Check sheet for the modelled part. Datum: model origin and axes. Units: mm. Face numbers are marked on the shaded views. A direction names the side the tool comes from. Give positions to 0.01 mm unless a question says otherwise; leave off trailing zeros. Loops run counter-clockwise (first coordinate to the right, second up) from the corner with the lowest first, then second, coordinate; pieces in that order, holes last. Notation, with made-up numbers: (73.25, 79) - (120.25, 79) arc R19 ccw to (120.25, 90) - close; hole circle Ø9 at (8.25, -36.5). An arc over 180 degrees is marked (long way). Use one line per item in the form item = value.
from build123d import *

# Parameters (mm, degrees)
SKETCH_1_R          = 4.1
SKETCH_1_R_2        = 1.6
EXTRUDE_1_DEPTH     = 7.5
CUT_EXTRUDE_1_DEPTH = 2.5
SKETCH_4_R          = 3.6
SKETCH_4_R_2        = 1.6
EXTRUDE_2_DEPTH     = 20
SKETCH_5_R          = 7
SKETCH_5_R_2        = 1.6
EXTRUDE_3_DEPTH     = 10
CUT_EXTRUDE_START   = -6.5
CUT_EXTRUDE_2_DEPTH = 6.5
SKETCH_7_R          = 1.6
CUT_EXTRUDE_3_DEPTH = 86.794813363
CHAMFER_1_SIZE      = 1
CHAMFER_1_SIZE_2    = 22
SKETCH_9_R          = 3.35
CUT_EXTRUDE_4_DEPTH = 3
SKETCH_11_R         = 3.35
CUT_EXTRUDE_5_DEPTH = 3


with BuildPart() as part:
    # 草图1 → 凸台-拉伸1 (new body)
    with BuildSketch(Plane.XY):
        Polygon((0, 11.5), (0, 4.5), (0.416202301, 4.5), (28, 4.5), (28, 0), (47, 0), (47, 4.5), (75, 4.5), (75, 18.5), (47, 18.5), (47, 23.5), (28, 23.5), (28, 18.5), (0, 18.5), align=None)
        with Locations((37.5, 11.5)):
            Circle(SKETCH_1_R, mode=Mode.SUBTRACT)
        with Locations((67.5, 11.5)):
            Circle(SKETCH_1_R_2, mode=Mode.SUBTRACT)
        with Locations((32.500024738, 3.227756818)):
            Circle(SKETCH_1_R_2, mode=Mode.SUBTRACT)
        with Locations((42.5, 3.25)):
            Circle(SKETCH_1_R_2, mode=Mode.SUBTRACT)
        with Locations((42.5, 19.75)):
            Circle(SKETCH_1_R_2, mode=Mode.SUBTRACT)
        with Locations((32.500024738, 19.75)):
            Circle(SKETCH_1_R_2, mode=Mode.SUBTRACT)
        with Locations((7.5, 11.5)):
            Circle(SKETCH_1_R_2, mode=Mode.SUBTRACT)
        with Locations((52.370486737, 11.554033831)):
            Circle(SKETCH_1_R_2, mode=Mode.SUBTRACT)
        with Locations((22.5, 11.5)):
            Circle(SKETCH_1_R_2, mode=Mode.SUBTRACT)
    extrude(amount=EXTRUDE_1_DEPTH)

    # 草图2 → 切除-拉伸1 (cut)
    with BuildSketch(Plane(origin=(0, 0, 0), x_dir=(-1, 0, 0), z_dir=(0, 0, -1))):
        Polygon((-38.862693304, 19.75), (-40.681346652, 22.9), (-44.318653348, 22.9), (-46.137306696, 19.75), (-44.318653348, 16.6), (-40.681346652, 16.6), align=None)
        Polygon((-28.862718042, 19.75), (-30.68137139, 22.9), (-34.318678086, 22.9), (-36.137331434, 19.75), (-34.318678086, 16.6), (-30.68137139, 16.6), align=None)
        Polygon((-38.862693304, 3.25), (-40.681346652, 6.4), (-44.318653348, 6.4), (-46.137306696, 3.25), (-44.318653348, 0.1), (-40.681346652, 0.1), align=None)
        Polygon((-28.862718042, 3.227756818), (-30.68137139, 6.377756818), (-34.318678086, 6.377756818), (-36.137331434, 3.227756818), (-34.318678086, 0.077756818), (-30.68137139, 0.077756818), align=None)
        Polygon((-63.862693304, 11.5), (-65.681346652, 14.65), (-69.318653348, 14.65), (-71.137306696, 11.5), (-69.318653348, 8.35), (-65.681346652, 8.35), align=None)
        Polygon((-3.862693304, 11.5), (-5.681346652, 14.65), (-9.318653348, 14.65), (-11.137306696, 11.5), (-9.318653348, 8.35), (-5.681346652, 8.35), align=None)
    extrude(amount=-CUT_EXTRUDE_1_DEPTH, mode=Mode.SUBTRACT)

    # 草图4 → 凸台-拉伸2 (add)
    # profile 1 of 2: a face of its own
    with BuildSketch(Plane.XY.offset(7.5)):
        with Locations(Location((7.5, 11.5, 0), (0, 0, 180))):
            Circle(SKETCH_4_R)
        with Locations(Location((7.5, 11.5, 0), (0, 0, 180))):
            Circle(SKETCH_4_R_2, mode=Mode.SUBTRACT)
    # profile 2 of 2: a face of its own
    with BuildSketch(Plane.XY.offset(7.5)):
        with Locations(Location((67.5, 11.5, 0), (0, 0, 180))):
            Circle(SKETCH_4_R)
        with Locations(Location((67.5, 11.5, 0), (0, 0, 180))):
            Circle(SKETCH_4_R_2, mode=Mode.SUBTRACT)
    extrude(amount=EXTRUDE_2_DEPTH)

    # 草图5 → 凸台-拉伸3 (add)
    # profile 1 of 2: a face of its own
    with BuildSketch(Plane.XY.offset(27.5)):
        with Locations((7.5, 11.5)):
            Circle(SKETCH_5_R)
        with Locations(Location((7.5, 11.5, 0), (0, 0, 180))):
            Circle(SKETCH_5_R_2, mode=Mode.SUBTRACT)
    # profile 2 of 2: a face of its own
    with BuildSketch(Plane.XY.offset(27.5)):
        with Locations((67.5, 11.5)):
            Circle(SKETCH_5_R)
        with Locations(Location((67.5, 11.5, 0), (0, 0, 180))):
            Circle(SKETCH_5_R_2, mode=Mode.SUBTRACT)
    extrude(amount=EXTRUDE_3_DEPTH)

    # 草图6 → 切除-拉伸2 (cut)
    with BuildSketch(Plane.XY.offset(37.5).offset(CUT_EXTRUDE_START)):
        with BuildLine():
            Line((1.5, 7.894448725), (1.5, 15.105551275))
            ThreePointArc((1.5, 15.105551275), (0.5, 11.5), (1.5, 7.894448725))
        make_face()
        with BuildLine():
            Line((73.5, 15.105551275), (73.5, 7.894448725))
            ThreePointArc((73.5, 7.894448725), (74.5, 11.5), (73.5, 15.105551275))
        make_face()
        with BuildLine():
            Line((3.5, 5.755437353), (3.5, 17.244562647))
            ThreePointArc((3.5, 17.244562647), (7.5, 18.5), (11.5, 17.244562647))
            Line((11.5, 17.244562647), (11.5, 5.755437353))
            ThreePointArc((11.5, 5.755437353), (7.5, 4.5), (3.5, 5.755437353))
        make_face()
        with BuildLine():
            Line((71.5, 7.894448725), (71.5, 17.244562647))
            ThreePointArc((71.5, 17.244562647), (67.5, 18.5), (63.5, 17.244562647))
            Line((63.5, 17.244562647), (63.5, 5.755437353))
            ThreePointArc((63.5, 5.755437353), (67.5, 4.5), (71.5, 5.755437353))
            Line((71.5, 5.755437353), (71.5, 7.894448725))
        make_face()
        with BuildLine():
            Line((13.5, 15.105551275), (13.5, 7.894448725))
            ThreePointArc((13.5, 7.894448725), (14.5, 11.5), (13.5, 15.105551275))
        make_face()
        with BuildLine():
            Line((61.5, 7.894448725), (61.5, 15.105551275))
            ThreePointArc((61.5, 15.105551275), (60.5, 11.5), (61.5, 7.894448725))
        make_face()
    extrude(amount=CUT_EXTRUDE_2_DEPTH, mode=Mode.SUBTRACT)

    # 草图7 → 切除-拉伸3 (cut, through all)
    with BuildSketch(Plane.ZY.offset(-1.5)):
        with Locations((34.25, 11.5)):
            Circle(SKETCH_7_R)
    extrude(amount=-CUT_EXTRUDE_3_DEPTH, mode=Mode.SUBTRACT)

    # 倒角1
    # the kernel refuses this chamfer: 22, 1 mm, written as the material it adds along each edge
    with BuildSketch(Plane(origin=(67.5, 11.5, 7.5), x_dir=(-1, 0, 0), z_dir=(0, 1, 0))) as chamfer_1_piece_1:
        Polygon((3.6 + CHAMFER_1_SIZE, 0), (3.6, CHAMFER_1_SIZE_2), (3.6, 0), align=None)
    revolve(axis=Axis((67.5, 11.5, 7.5), (0, 0, 1)))
    with BuildSketch(Plane(origin=(7.5, 11.5, 7.5), x_dir=(-1, 0, 0), z_dir=(0, 1, 0))) as chamfer_1_piece_2:
        Polygon((3.6 + CHAMFER_1_SIZE, 0), (3.6, CHAMFER_1_SIZE_2), (3.6, 0), align=None)
    revolve(axis=Axis((7.5, 11.5, 7.5), (0, 0, 1)))

    # 草图9 → 切除-拉伸4 (cut)
    with BuildSketch(Plane.XY.offset(31)):
        with Locations((7.5, 11.5)):
            Circle(SKETCH_9_R)
    extrude(amount=-CUT_EXTRUDE_4_DEPTH, mode=Mode.SUBTRACT)

    # 草图11 → 切除-拉伸5 (cut)
    with BuildSketch(Plane.XY.offset(31)):
        with Locations((67.5, 11.5)):
            Circle(SKETCH_11_R)
    extrude(amount=-CUT_EXTRUDE_5_DEPTH, mode=Mode.SUBTRACT)


solid = part.part
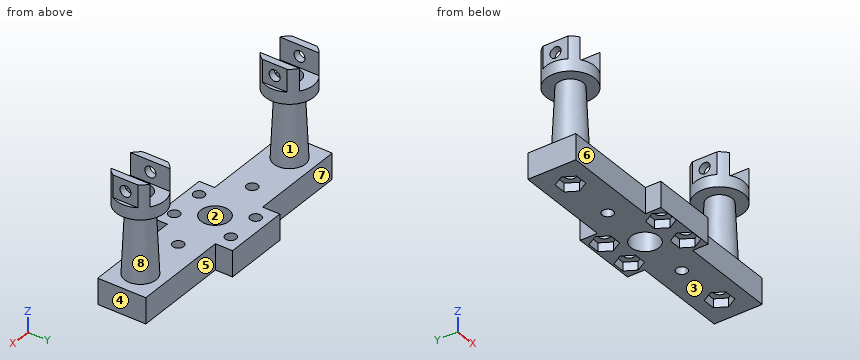
Item 1: Access from +Z, -Z, +X, -X, +Y, -Y to the whole of each face (thin tool, end or side, straight path). Record for the marked faces 5, 6, 7 and 8.
Answer block:
face_5 = +Z, -Z, +X, +Y
face_6 = +Z, -Z, -X, -Y
face_7 = +Z, -Z, -X, +Y
face_8 = none
Item 2: Thickness scan on L1, parallel to Y at x = 42.5, z = 4.2; L2, parallel to X at y = 5.75, z = 28; L3, parallel to Y at x = 37.5, z = 5.25. Record the ranges inside material, lowest first.
Answer block:
L1 = 0 to 1.65, 4.85 to 18.15, 21.35 to 23.5
L2 = 3.51 to 11.49, 63.51 to 71.49
L3 = 0 to 7.4, 15.6 to 23.5
Item 3: Mould release check, pull along X, two halves, no side actions. Record for the marked faces 1, 2, 3 and 4: released by +X, released by -X, zero draft, split by the parting line, or undercut.
Answer block:
face_1 = undercut
face_2 = undercut
face_3 = zero draft
face_4 = released by +X
Item 4: Gauge pin test, flat ends, axial feed: P1, Ø10, axis at y = 12.5, z = 16, coming from the +X side; P2, Ø0.8, axis at x = 8.5, z = 2, coming from the +Y side; P3, Ø1, axis at x = 20, y = 11, coming from the +Z side. Record the tip position at first contact, or that the pin passes through.
Answer block:
P1 = 71.94
P2 = 18.5
P3 = 7.5
Item 5: Section check A-A on x = 37.5. Record the boundary of the cut face in (y, z).
Answer block:
outline = (0, 0) - (7.4, 0) - (7.4, 7.5) - (0, 7.5) - close; (15.6, 0) - (23.5, 0) - (23.5, 7.5) - (15.6, 7.5) - close
Item 6: Section check B-B on z = 34.25. Give the number of separate pieces and of enclosed holes in the cut face, then the cut area to 3 significant figures.
Answer block:
separate_pieces = 8
enclosed_holes = 0
area = 51.6 mm2
Item 7: Section check C-C on z = 13. Record the boundary of the cut face in (x, y), then the cut area to 3 significant figures.
Answer block:
outline = circle Ø8.7 at (7.5, 11.5); circle Ø8.7 at (67.5, 11.5); hole circle Ø3.2 at (7.5, 11.5); hole circle Ø3.2 at (67.5, 11.5)
area = 103 mm2
Item 8: Section check D-D on x = 59.5. Record the boundary of the cut face in (y, z).
Answer block:
outline = (4.5, 0) - (18.5, 0) - (18.5, 7.5) - (4.5, 7.5) - close
